Check sheet for the modelled part. Datum: model origin and axes. Units: mm. Round coordinates to 2 decimals unless told otherwise and drop trailing zeros. Write each loop counter-clockwise with the first axis right and the second up, starting at its lowest first coordinate (ties: lowest second). Pieces come first, ordered by that corner, then holes. Notation, with made-up numbers: (-38.75, 1.25) -> (-34.75, 1.25) arc R24 ccw to (-34.75, 14.25) -> close; hole circle Ø11 at (22.25, 61.25). An arc over 180 degrees is marked (long way). One line per item, written item: value.
from build123d import *

# Parameters (mm, degrees)
F0_W     = 1600
F0_H     = 300
F1_DEPTH = 1.5


with BuildPart() as f1:
    # F0 (on Front) → F1 (new body, symmetric)
    with BuildSketch(Plane.XZ):
        Rectangle(F0_W, F0_H)
        with BuildLine():
            Line((-315, 80), (-315, 0))
            Line((-315, 0), (-315, -80))
            ThreePointArc((-315, -80), (-311.4644660941, -81.4644660941), (-310, -85))
            ThreePointArc((-310, -85), (-315, -90), (-320, -85))
            Line((-320, -85), (-400, -85))
            Line((-400, -85), (-480, -85))
            ThreePointArc((-480, -85), (-488.5355339059, -88.5355339059), (-485, -80))
            Line((-485, -80), (-485, -5.63e-07))
            Line((-485, -5.63e-07), (-485, 80))
            ThreePointArc((-485, 80), (-488.5355339059, 88.5355339059), (-480, 85))
            Line((-480, 85), (-400, 85))
            Line((-400, 85), (-320, 85))
            ThreePointArc((-320, 85), (-315, 90), (-310, 85))
            ThreePointArc((-310, 85), (-311.4644660941, 81.4644660941), (-315, 80))
        make_face(mode=Mode.SUBTRACT)
        with BuildLine():
            Line((485, 80), (485, 0))
            Line((485, 0), (485, -80))
            ThreePointArc((485, -80), (488.5355339059, -81.4644660941), (490, -85))
            ThreePointArc((490, -85), (485, -90), (480, -85))
            Line((480, -85), (400, -85))
            Line((400, -85), (320, -85))
            ThreePointArc((320, -85), (311.4644660941, -88.5355339059), (315, -80))
            Line((315, -80), (315, -5.63e-07))
            Line((315, -5.63e-07), (315, 80))
            ThreePointArc((315, 80), (311.4644660941, 88.5355339059), (320, 85))
            Line((320, 85), (400, 85))
            Line((400, 85), (480, 85))
            ThreePointArc((480, 85), (485, 90), (490, 85))
            ThreePointArc((490, 85), (488.5355339059, 81.4644660941), (485, 80))
        make_face(mode=Mode.SUBTRACT)
        with BuildLine():
            ThreePointArc((-485, -5.63e-07), (-460.1040765999, 60.1040762018), (-400, 85))
            Line((-400, 85), (-480, 85))
            ThreePointArc((-480, 85), (-481.4644660941, 81.4644660941), (-485, 80))
            Line((-485, 80), (-485, -5.63e-07))
        make_face()
        with BuildLine():
            ThreePointArc((-400, 85), (-339.8959235991, 60.1040764009), (-315, 0))
            Line((-315, 0), (-315, 80))
            ThreePointArc((-315, 80), (-318.5355339059, 81.4644660941), (-320, 85))
            Line((-320, 85), (-400, 85))
        make_face()
        with BuildLine():
            Line((-480, -85), (-400, -85))
            ThreePointArc((-400, -85), (-460.1040762018, -60.1040765999), (-485, -5.63e-07))
            Line((-485, -5.63e-07), (-485, -80))
            ThreePointArc((-485, -80), (-481.4644660941, -81.4644660941), (-480, -85))
        make_face()
        with BuildLine():
            Line((-315, -80), (-315, 0))
            ThreePointArc((-315, 0), (-339.8959235991, -60.1040764009), (-400, -85))
            Line((-400, -85), (-320, -85))
            ThreePointArc((-320, -85), (-318.5355339059, -81.4644660941), (-315, -80))
        make_face()
        with BuildLine():
            ThreePointArc((315, -5.63e-07), (339.8959234001, 60.1040762018), (400, 85))
            Line((400, 85), (320, 85))
            ThreePointArc((320, 85), (318.5355339059, 81.4644660941), (315, 80))
            Line((315, 80), (315, -5.63e-07))
        make_face()
        with BuildLine():
            ThreePointArc((400, 85), (460.1040764009, 60.1040764009), (485, 0))
            Line((485, 0), (485, 80))
            ThreePointArc((485, 80), (481.4644660941, 81.4644660941), (480, 85))
            Line((480, 85), (400, 85))
        make_face()
        with BuildLine():
            Line((320, -85), (400, -85))
            ThreePointArc((400, -85), (339.8959237982, -60.1040765999), (315, -5.63e-07))
            Line((315, -5.63e-07), (315, -80))
            ThreePointArc((315, -80), (318.5355339059, -81.4644660941), (320, -85))
        make_face()
        with BuildLine():
            Line((485, -80), (485, 0))
            ThreePointArc((485, 0), (460.1040764009, -60.1040764009), (400, -85))
            Line((400, -85), (480, -85))
            ThreePointArc((480, -85), (481.4644660941, -81.4644660941), (485, -80))
        make_face()
    extrude(amount=F1_DEPTH, both=True)


solid = f1.part
Item 1: Thickness scan on line 1 (Z direction, x = 372, y = 0.8); line 2 (X direction, y = 0.85, z = 26); line 3 (Z direction, x = -335.5, y = -1). Record the ranges inside material, lowest first.
Answer:
line 1: z = -150 to -80.26, 80.26 to 150
line 2: x = -800 to -480.93, -319.07 to 319.07, 480.93 to 800
line 3: z = -150 to -55.36, 55.36 to 150
Item 2: Depth check by flat-ended pin: P1, Ø6, axis at x = 315, z = 85, coming from the -Y side. Enter the tip coordinate at first touch or a pass-through.
Answer:
P1: passes through
Item 3: Sectioned sample at B-B on z = -47.5. Enter the section's corners in (x, y), and give its area (3 significant figures).
Answer:
outline: (-800, -1.5) -> (-470.49, -1.5) -> (-470.49, 1.5) -> (-800, 1.5) -> close; (-329.51, -1.5) -> (329.51, -1.5) -> (329.51, 1.5) -> (-329.51, 1.5) -> close; (470.49, -1.5) -> (800, -1.5) -> (800, 1.5) -> (470.49, 1.5) -> close
area: 3,950 mm^2
Item 4: Sectioned sample at A-A on y = -0.95. Count the separate pieces of the cut face and the enclosed holes in it, and give its area (3 significant figures).
Answer:
separate pieces: 1
enclosed holes: 10
area: 434,000 mm^2
